```python
from build123d import *

# Parameters (mm, degrees)
F1_DEPTH        = 10
F5_R            = 2
F6_W            = 50
F6_H            = 45
F7_DEPTH        = 20
F10_D           = 2
F10_DEPTH       = 20
F10_CSINK_D     = 10
F10_CSINK_ANGLE = 82
F10_TIP         = 0.600860619
F11_R           = 5
F12_R           = 1.75
F13_DEPTH       = 5
F15_W           = 33.0769233406
F15_H           = 100.1923158765
F16_DEPTH       = 50.001
F17_R           = 1.825
F18_DEPTH       = 6


with BuildPart() as f1:
    # F0 (on Right) → F1 (new body, symmetric)
    with BuildSketch(Plane.YZ):
        with BuildLine():
            Line((-15, 0), (0, 0))
            Line((0, 0), (0, 24.5))
            Line((0, 24.5), (-5, 24.5))
            ThreePointArc((-5, 24.5), (-11.3675088396, 12.8081668733), (-15, 0))
        make_face()
    extrude(amount=F1_DEPTH, both=True)

    # F3 (on Right) → F4 (revolve)
    with BuildSketch(Plane.YZ):
        Polygon((0, 12.25), (15, 12.25), (15, 13.75), (10, 13.75), (1.75, 16.75), (1.75, 15.5), (0, 15.5), align=None)
    revolve(axis=Axis((0, 7.5, 12.25), (0, -1, 0)))

    # F5
    f5_edges = [f1.edges().sort_by_distance(p)[0] for p in [
        (0, -5, 24.5),
        (0, -15, 0),
        (0, 0, 0),
    ]]
    fillet(f5_edges, radius=F5_R)


with BuildPart() as f7:
    # F6 (on Right) → F7 (new body)
    with BuildSketch(Plane.YZ):
        with Locations((0, 10)):
            Rectangle(F6_W, F6_H)
    extrude(amount=F7_DEPTH)

    # F8: cut F1
    add(f1.part, mode=Mode.SUBTRACT)

    # F10
    with Locations(Plane.XZ.offset(25)):
        with Locations((0, 12.25)):
            CounterSinkHole(F10_D / 2, F10_CSINK_D / 2, depth=F10_DEPTH, counter_sink_angle=F10_CSINK_ANGLE)
            with Locations((0, 0, -(F10_DEPTH + F10_TIP / 2))):  # 118° drill point
                Cone(0, F10_D / 2, F10_TIP, mode=Mode.SUBTRACT)

    # F11
    f11_edges = [f7.edges().sort_by_distance(p)[0] for p in [
        (10, -25, 32.5),
        (10, 25, 32.5),
        (10, -25, -12.5),
        (10, 25, -12.5),
    ]]
    fillet(f11_edges, radius=F11_R)

    # F12 (on face) → F13 (join)
    with BuildSketch(Plane.YZ):
        with Locations((20, 27.5)):
            Circle(F12_R)
        with Locations((-20, 27.5)):
            Circle(F12_R)
        with Locations((-20, -7.5)):
            Circle(F12_R)
        with Locations((20, -7.5)):
            Circle(F12_R)
    extrude(amount=-F13_DEPTH)

    # F14: F7 across plane


with BuildPart() as f7_1:
    add(f7.part)
    add(f7.part.mirror(Plane.YZ))

    # F15 (on face) → F16 (cut, through all)
    with BuildSketch(Plane.XZ.offset(25)):
        with Locations((16.5384616703, 1.5384629369)):
            Rectangle(F15_W, F15_H)
    extrude(amount=-F16_DEPTH, mode=Mode.SUBTRACT)

    # F17 (on face) → F18 (cut)
    with BuildSketch(Plane.YZ):
        with Locations((-20, 27.5)):
            Circle(F17_R)
        with Locations((20, 27.5)):
            Circle(F17_R)
        with Locations((20, -7.5)):
            Circle(F17_R)
        with Locations((-20, -7.5)):
            Circle(F17_R)
    extrude(amount=-F18_DEPTH, mode=Mode.SUBTRACT)


solid = f7_1.part
```
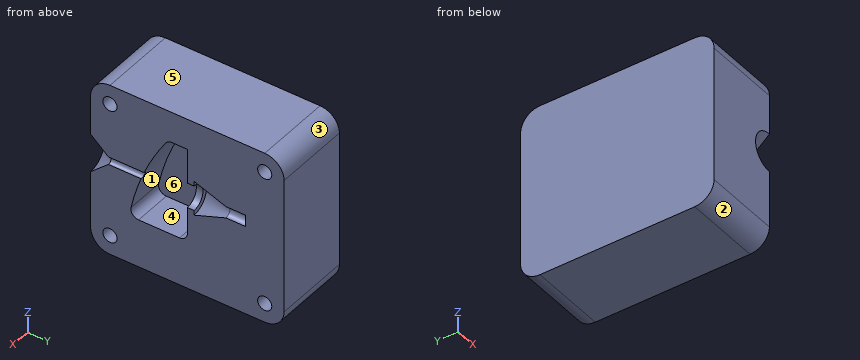
The model under review builds one solid part; all positions refer to its coordinate system, in mm. Face numbers are marked on the shaded views. A direction names the side the tool comes from. Round coordinates to 2 decimals unless told otherwise and drop trailing zeros. Order: outer loops, then holes, each group sorted by start corner. A loop starts at its lowest first (then second) coordinate and runs counter-clockwise, first axis right, second up.
(1) Tool access review of the marked faces 5 and 6: name each direction out of +Z, -Z, +X, -X, +Y, -Y from which nothing blocks a thin tool from reaching the whole face with its end or side.
Working result:
face 5: +Z, +X, -X, +Y, -Y
face 6: +X
(2) Take a section at A-A, the plane y = -3. State the section outline as (x, z) points, plus the area to 3 significant figures.
Working result:
outline: (-20, -12.5) - (0, -12.5) - (0, 0) - (-10, 0) - (-10, 24.5) - (0, 24.5) - (0, 32.5) - (-20, 32.5) - close
area: 655 mm2
(3) Take a section at C-C, the plane z = 6.5. State the section outline as (x, y) points, plus the area to 3 significant figures.
Working result:
outline: (-20, -25) - (0, -25) - (0, -13.54) - (-10, -13.54) - (-10, 0) - (0, 0) - (0, 25) - (-20, 25) - close
area: 865 mm2
(4) Take a section at B-B, the plane z = 12.25. State the section outline as (x, y) points.
Working result:
outline: (-20, -25) - (-5, -25) - (-1, -20.4) - (-1, -11.59) - (-10, -11.59) - (-10, 0) - (-3.25, 0) - (-3.25, 1.75) - (-4.5, 1.75) - (-1.5, 10) - (-1.5, 15) - (0, 15) - (0, 25) - (-20, 25) - close
(5) Wall thickness on L1, parallel to Z at x = -2.3, y = -20 (3 decimals); L2, parallel to X at y = -9, z = 8.5; L3, parallel to Y at x = -2, z = 1: over which ranges is each line inside the solid? List them lowest first.
Working result:
L1: z = -12.5 to -9.325, -5.675 to 25.675, 29.325 to 32.5
L2: x = -20 to -10
L3: y = -25 to -14.32, -0.27 to 25
(6) For P1, Ø1.1, axis at y = 20.5, z = 26.5, coming from the +X side; P2, Ø1.6, axis at x = -0.5, z = 13, coming from the -Y side; P3, Ø3, axis at y = 1, z = 12, coming from the +X side, all flat-tipped, find the tip position at first contact; note any pin that passes through.
Working result:
P1: stops at x = -6
P2: stops at y = -21.21
P3: stops at x = -2.74
(7) Mouldability with a two-part tool opening along Y and no side actions: class the marked faces 1, 2, 3 and 4 as released by +Y, released by -Y, zero draft, split by the parting line, or undercut.
Working result:
face 1: undercut
face 2: released by -Y
face 3: released by +Y
face 4: undercut
